The drawing under review shows one solid part. Ordinate dimensions are in mm from its lowest x, y, z. A direction names the side the tool comes from. Coordinates: 2 decimals unless noted, no trailing zeros. Write each loop counter-clockwise with the first axis right and the second up, starting at its lowest first coordinate (ties: lowest second). Pieces come first, ordered by that corner, then holes.
1) To check wall thickness, follow line 1 along Z through (x, y) = (7.5, 15.3); line 2 along X through (y, z) = (18.25, 6.75); line 3 along X through (y, z) = (14, 4.5) (1 decimal). State the ranges of each line that lie inside material, in increasing order.
2) We need section B-B on x = 68.5. Write out the cut boundary in (y, z).
3) Mouldability with a two-part tool opening along X and no side actions: class the marked faces 1, 2 and 3 as pulls with the +X half, pulls with the -X half, needs draft (parallel to the pull), parting line crosses it, or undercut.
4) We need section C-C on y = 17. Write out the cut boundary in (x, z), then the cut area to 3 significant figures.
5) Insertion check: P1, Ø4, axis at x = 27.5, z = 6, coming from the -Y side; P2, Ø5.5, axis at x = 7.5, z = 5, coming from the +Y side; P3, Ø5, axis at x = 67, z = 4.5, coming from the -Y side; P4, Ø4, axis at x = 68.5, z = 5, coming from the +Y side. Each pin has a flat end and moves straight along its axis. Give the tip position at first contact, or say it passes through.
6) For the marked faces 4 and 5, list the 3-axis set-ups (+Z, -Z, +X, -X, +Y, -Y) from which the entire face can be reached by the end or side of a thin tool; tool diameter is ignored.
7) We need section A-A on z = 5. Give the number of separate pieces and of enclosed holes in the cut face, then the cut area to 3 significant figures.
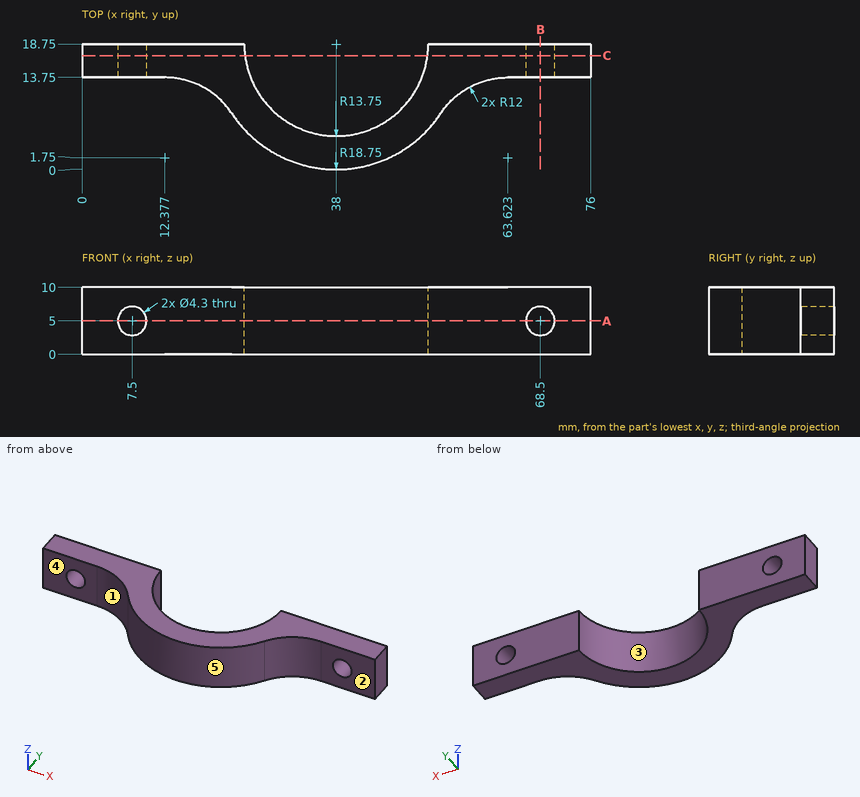
Result:
1. line 1: z = 0 to 2.85, 7.15 to 10
1. line 2: x = 0 to 6.25, 8.75 to 24.26, 51.74 to 67.25, 69.75 to 76
1. line 3: x = 0 to 5.4, 9.6 to 25.1, 50.9 to 66.4, 70.6 to 76
2. outline: (13.75, 0) - (18.75, 0) - (18.75, 2.85) - (13.75, 2.85) - close; (13.75, 7.15) - (18.75, 7.15) - (18.75, 10) - (13.75, 10) - close
3. face 1: pulls with the -X half
3. face 2: needs draft
3. face 3: undercut
4. outline: (0, 0) - (24.36, 0) - (24.36, 10) - (0, 10) - close; (51.64, 0) - (76, 0) - (76, 10) - (51.64, 10) - close; hole circle Ø4.3 at (7.5, 5); hole circle Ø4.3 at (68.5, 5)
4. area: 458 mm2
5. P1: stops at y = 2.04
5. P2: stops at y = 18.75
5. P3: stops at y = 13.75
5. P4: passes through
6. face 4: +Z, -Z, -X, -Y
6. face 5: +Z, -Z, -Y
7. separate pieces: 3
7. enclosed holes: 0
7. area: 424 mm2
